Can you work these out from the model? Positions are in its coordinate system, mm. A direction names the side the tool comes from. Coordinates: 2 decimals unless noted, no trailing zeros. Order: outer loops, then holes, each group sorted by start corner. A loop starts at its lowest first (then second) coordinate and runs counter-clockwise, first axis right, second up. Notation, with made-up numbers: (-39, 51.5) -> (-21, 51.5) arc R19 cw to (-21, 70.5) -> close; hole circle Ø11 at (75, 83). An arc over 180 degrees is marked (long way). Write item = value, one per line.
```python
from build123d import *

# Parameters (mm, degrees)
SKETCH1_W           = 54
SKETCH1_H           = 90
SKETCH1_W_2         = 38
SKETCH1_H_2         = 74
BOSS_EXTRUDE1_DEPTH = 30
CUT_EXTRUDE1_DEPTH  = 4.1
SKETCH5_R           = 4.1
CUT_EXTRUDE2_DEPTH  = 0.5
CUT_EXTRUDE3_DEPTH  = 4.1
SKETCH7_R           = 4.1
CUT_EXTRUDE4_DEPTH  = 0.5
SKETCH8_W           = 54
SKETCH8_H           = 90
BOSS_EXTRUDE2_DEPTH = 2
SKETCH9_W           = 54
SKETCH9_H           = 90
BOSS_EXTRUDE3_DEPTH = 2
SKETCH10_W          = 54
SKETCH10_H          = 90
CUT_EXTRUDE5_DEPTH  = 17
SKETCH11_R          = 17.5
CUT_EXTRUDE6_DEPTH  = 3
CUT_EXTRUDE7_DEPTH  = 18
CUT_EXTRUDE8_DEPTH  = 5
FILLET1_R           = 5


with BuildPart() as part:
    # Sketch1 → Boss-Extrude1 (new body)
    with BuildSketch(Plane.XY):
        with Locations((27, 45)):
            Rectangle(SKETCH1_W, SKETCH1_H)
        with Locations((27, 45)):
            Rectangle(SKETCH1_W_2, SKETCH1_H_2, mode=Mode.SUBTRACT)
    extrude(amount=BOSS_EXTRUDE1_DEPTH)

    # Sketch2 → Cut-Extrude1 (cut)
    with BuildSketch(Plane.ZY.offset(-46)):
        Polygon((20.888972746, 65.4), (17.944486373, 70.5), (12.055513627, 70.5), (9.111027254, 65.4), (12.055513627, 60.3), (17.944486373, 60.3), align=None)
        Polygon((20.888972746, 24.6), (17.944486373, 29.7), (12.055513627, 29.7), (9.111027254, 24.6), (12.055513627, 19.5), (17.944486373, 19.5), align=None)
    extrude(amount=-CUT_EXTRUDE1_DEPTH, mode=Mode.SUBTRACT)

    # Sketch5 → Cut-Extrude2 (cut)
    with BuildSketch(Plane.ZY.offset(-50.1)):
        with Locations((15, 65.4)):
            Circle(SKETCH5_R)
        with Locations((15, 24.6)):
            Circle(SKETCH5_R)
    extrude(amount=-CUT_EXTRUDE2_DEPTH, mode=Mode.SUBTRACT)

    # Sketch6 → Cut-Extrude3 (cut)
    with BuildSketch(Plane(origin=(8, 0, 0), x_dir=(0, 0, -1), z_dir=(1, 0, 0))):
        Polygon((-9.111027254, 65.4), (-12.055513627, 70.5), (-17.944486373, 70.5), (-20.888972746, 65.4), (-17.944486373, 60.3), (-12.055513627, 60.3), align=None)
        Polygon((-9.111027254, 24.6), (-12.055513627, 29.7), (-17.944486373, 29.7), (-20.888972746, 24.6), (-17.944486373, 19.5), (-12.055513627, 19.5), align=None)
    extrude(amount=-CUT_EXTRUDE3_DEPTH, mode=Mode.SUBTRACT)

    # Sketch7 → Cut-Extrude4 (cut)
    with BuildSketch(Plane(origin=(3.9, 0, 0), x_dir=(0, 0, -1), z_dir=(1, 0, 0))):
        with Locations((-15, 65.4)):
            Circle(SKETCH7_R)
        with Locations((-15, 24.6)):
            Circle(SKETCH7_R)
    extrude(amount=-CUT_EXTRUDE4_DEPTH, mode=Mode.SUBTRACT)

    # Sketch8 → Boss-Extrude2 (add)
    with BuildSketch(Plane.XY.offset(30)):
        with Locations((27, 45)):
            Rectangle(SKETCH8_W, SKETCH8_H)
    extrude(amount=BOSS_EXTRUDE2_DEPTH)

    # Sketch9 → Boss-Extrude3 (add)
    with BuildSketch(Plane(origin=(0, 0, 0), x_dir=(-1, 0, 0), z_dir=(0, 0, -1))):
        with Locations((-27, 45)):
            Rectangle(SKETCH9_W, SKETCH9_H)
    extrude(amount=BOSS_EXTRUDE3_DEPTH)

    # Sketch10 → Cut-Extrude5 (cut)
    with BuildSketch(Plane.XY.offset(32)):
        with Locations((27, 45)):
            Rectangle(SKETCH10_W, SKETCH10_H)
    extrude(amount=-CUT_EXTRUDE5_DEPTH, mode=Mode.SUBTRACT)

    # Sketch11 → Cut-Extrude6 (cut, through all)
    with BuildSketch(Plane.XY):
        with Locations((27, 45)):
            Circle(SKETCH11_R)
    extrude(amount=-CUT_EXTRUDE6_DEPTH, mode=Mode.SUBTRACT)

    # Sketch12 → Cut-Extrude7 (cut, through all)
    with BuildSketch(Plane.XY.offset(15)):
        Polygon((5.443375673, 86), (4.721687836, 87.25), (3.278312164, 87.25), (2.556624327, 86), (3.278312164, 84.75), (4.721687836, 84.75), align=None)
        Polygon((51.443375673, 86), (50.721687836, 87.25), (49.278312164, 87.25), (48.556624327, 86), (49.278312164, 84.75), (50.721687836, 84.75), align=None)
        Polygon((3.278312164, 2.75), (4.721687836, 2.75), (5.443375673, 4), (4.721687836, 5.25), (3.278312164, 5.25), (2.556624327, 4), align=None)
        Polygon((50.721687836, 5.25), (49.278312164, 5.25), (48.556624327, 4), (49.278312164, 2.75), (50.721687836, 2.75), (51.443375673, 4), align=None)
    extrude(amount=-CUT_EXTRUDE7_DEPTH, mode=Mode.SUBTRACT)

    # Sketch13 → Cut-Extrude8 (cut)
    with BuildSketch(Plane(origin=(0, 90, 0), x_dir=(1, 0, 0), z_dir=(0, 1, 0))):
        Polygon((10, -2.556624327), (8.75, -3.278312164), (8.75, -4.721687836), (10, -5.443375673), (11.25, -4.721687836), (11.25, -3.278312164), align=None)
        Polygon((44, -2.556624327), (42.75, -3.278312164), (42.75, -4.721687836), (44, -5.443375673), (45.25, -4.721687836), (45.25, -3.278312164), align=None)
    extrude(amount=-CUT_EXTRUDE8_DEPTH, mode=Mode.SUBTRACT)

    # Fillet1
    fillet1_edges = [part.edges().sort_by_distance(p)[0] for p in [
        (0, 0, 6.5),
        (54, 0, 6.5),
    ]]
    fillet(fillet1_edges, radius=FILLET1_R)


solid = part.part
```
Item 1: For faces 4 (the flat face through (27, 90, 7)), 5 (the flat face through (8, 44, 7)), which set-ups out of +Z, -Z, +X, -X, +Y, -Y let a thin tool reach every point of the face, with its end or its side?
A:
face_4 = +Z, -Z, +X, -X, +Y
face_5 = +Z
Item 2: If we mould it in two halves opening along Y, with no side actions, what happens to faces 1 (the flat face through (3.4, 65, 13)), 2 (the cylindrical face through (53, 2, 6)), 3 (the flat face through (44, 85, 4))? For each: pulls with the +Y half, pulls with the -Y half, needs draft (parallel to the pull), parting line crosses it, or undercut.
A:
face_1 = undercut
face_2 = pulls with the -Y half
face_3 = pulls with the +Y half
Item 3: I want a section at C-C, the plane x = 27. Please give me the cut outline in (y, z).
A:
outline = (0, -2) -> (27.5, -2) -> (27.5, 0) -> (8, 0) -> (8, 15) -> (0, 15) -> close; (62.5, -2) -> (90, -2) -> (90, 15) -> (82, 15) -> (82, 0) -> (62.5, 0) -> close
Item 4: I'm going to push flat-ended pins straight in: P1, Ø1.5, axis at x = 10.5, y = 45.5, coming from the +Z side; P2, Ø1.2, axis at x = 49.5, z = 3, coming from the -Y side; P3, Ø10, axis at x = 32.5, y = 64, coming from the +Z side. Where does each tip first touch, or does it pass through?
A:
P1 = through
P2 = 0
P3 = 0
Item 5: If I drill on probe 1 along X at (y, z) = (43, 2.75); probe 2 along Y at (x, z) = (11.5, 12.25); probe 3 along Y at (x, z) = (27, -1.35), over which ranges is the centre line in solid material (lowest first)?
A:
probe_1 = 0 to 8, 46 to 54
probe_2 = 0 to 8, 82 to 90
probe_3 = 0 to 27.5, 62.5 to 90
Item 6: I want a section at B-B, the plane z = 7.5. Give the number of separate pieces and of enclosed holes in the cut face, plus the area to 3 significant figures.
A:
separate_pieces = 1
enclosed_holes = 5
area = 2,020 mm2
Item 7: I want a section at A-A, the plane y = 45. Please give me the cut outline in (x, z).
A:
outline = (0, -2) -> (9.5, -2) -> (9.5, 0) -> (8, 0) -> (8, 15) -> (0, 15) -> close; (44.5, -2) -> (54, -2) -> (54, 15) -> (46, 15) -> (46, 0) -> (44.5, 0) -> close
Item 8: I want a section at D-D, the plane y = 74.5. Please give me the cut outline in (x, z).
A:
outline = (0, -2) -> (54, -2) -> (54, 15) -> (46, 15) -> (46, 0) -> (8, 0) -> (8, 15) -> (0, 15) -> close
